Verification items for the finished model (mm, model axes). Face numbers are marked on the shaded views. A direction names the side the tool comes from. Round coordinates to 2 decimals unless told otherwise and drop trailing zeros. Write each loop counter-clockwise with the first axis right and the second up, starting at its lowest first coordinate (ties: lowest second). Pieces come first, ordered by that corner, then holes. Notation, with made-up numbers: M 54,-24 L 58,-24 A16 cw 58,3 Z; hole C 60,57.5 d1. An arc over 180 degrees is marked long. One line per question, with ' | ' between items.
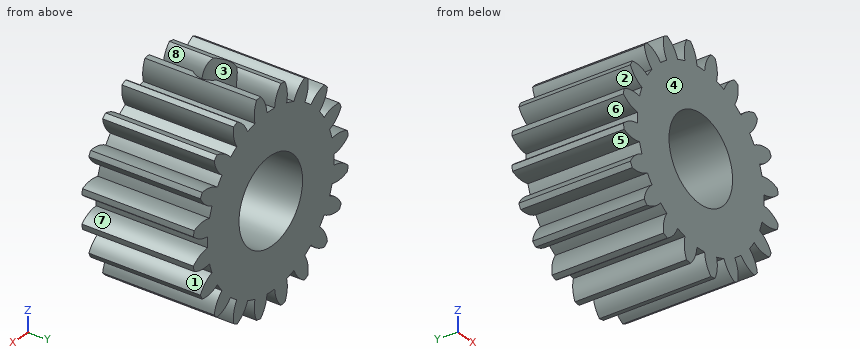
from build123d import *

# Parameters (mm, degrees)
SKETCH1_R                    = 11.684
BOSS_EXTRUDE1_DEPTH          = 12.7
F_3_8_0_375_DIAMETER_HOLE1_D = 9.525
CUT_EXTRUDE1_DEPTH           = 21.840386561
CIRPATTERN1_COUNT            = 20
F_10_32_TAPPED_HOLE2_REACH   = 30.849
F_10_32_TAPPED_HOLE2_BORE_R  = 2.0193


with BuildPart() as part:
    # Sketch1 → Boss-Extrude1 (new body)
    with BuildSketch(Plane(origin=(0, 0, 0), x_dir=(1, 0, 0), z_dir=(0, 1, 0))):
        with Locations(Location((0, 0, 0), (0, 0, 270))):
            Circle(SKETCH1_R)
    extrude(amount=BOSS_EXTRUDE1_DEPTH)

    # 3/8 (0.375) Diameter Hole1 (through all)
    with Locations(Plane(origin=(0, 12.7, 0), x_dir=(1, 0, 0), z_dir=(0, 1, 0))):
        with Locations((0, 0)):
            Hole(F_3_8_0_375_DIAMETER_HOLE1_D / 2)

    # Sketch6 → Cut-Extrude1 (cut, through all)
    with BuildSketch(Plane(origin=(0, 12.7, 0), x_dir=(1, 0, 0), z_dir=(0, 1, 0))):
        with BuildLine():
            ThreePointArc((-1.52506803, 11.58404176), (0, 11.684), (1.52506803, 11.58404176))
            ThreePointArc((1.52506803, 11.58404176), (0.859486594, 10.605826694), (0.578386073, 9.456528707))
            ThreePointArc((0.578386073, 9.456528707), (0, 9.4742), (-0.578386073, 9.456528707))
            ThreePointArc((-0.578386073, 9.456528707), (-0.859486594, 10.605826694), (-1.52506803, 11.58404176))
        make_face()
    cut_extrude1 = extrude(amount=-CUT_EXTRUDE1_DEPTH, mode=Mode.SUBTRACT)

    # CirPattern1: Cut-Extrude1 ×20 about axis
    cirpattern1_axis = Axis((0, 0, 0), (0, 1, 0))
    for i in range(1, CIRPATTERN1_COUNT):
        add(cut_extrude1.rotate(cirpattern1_axis, i * 360 / CIRPATTERN1_COUNT), mode=Mode.SUBTRACT)

    # #10-32 Tapped Hole2 bore → #10-32 Tapped Hole2 (cut, up to next)
    with BuildSketch(Plane.XY.offset(11.58404176), mode=Mode.PRIVATE) as f_10_32_tapped_hole2_sk1:
        with Locations((0, 6.35)):
            Circle(F_10_32_TAPPED_HOLE2_BORE_R)
    f_10_32_tapped_hole2_tool1 = extrude(f_10_32_tapped_hole2_sk1.sketch, amount=-F_10_32_TAPPED_HOLE2_REACH, mode=Mode.PRIVATE) & part.part
    add(f_10_32_tapped_hole2_tool1.solids().sort_by_distance((0, 6.35, 11.584042))[0], mode=Mode.SUBTRACT)


solid = part.part
1. Go/stop test with flat-tipped pins: P1, Ø10, axis at x = 2, z = -1, coming from the +Y side; P2, Ø5.5, axis at x = 0, y = 6.35, coming from the -Z side; P3, Ø4, axis at y = 2, z = 8, coming from the +X side; P4, Ø1, axis at y = 4.5, z = 6, coming from the -X side. Record where each tip stops, or that it passes through.
Results:
P1: stops at y = 12.7 | P2: stops at z = -11.58 | P3: stops at x = 8.48 | P4: stops at x = -10.31
2. Section check C-C, the plane z = -3. Record the cut outline in (x, y).
Results:
outline: M -8.99,0 L -3.7,0 L -3.7,12.7 L -8.99,12.7 Z; M 3.7,0 L 8.99,0 L 8.99,12.7 L 3.7,12.7 Z
3. Tool access check on the marked faces 5, 6, 7 and 8. Record the directions out of +Z, -Z, +X, -X, +Y, -Y that give a thin tool (end or side, any length) a straight path to the whole face; none if there is none.
Results:
face 5: +Y, -Y | face 6: -X, +Y, -Y | face 7: +X, +Y, -Y | face 8: +Z, +Y, -Y
4. Thickness scan on line 1 (Z direction, x = 0, y = 4); line 2 (X direction, y = 6.35, z = 9.5); line 3 (Z direction, x = -9.25, y = 6). Record the ranges inside material, lowest first.
Results:
line 1: z = -9.47 to -4.76, 4.76 to 9.47 | line 2: x = -5.6 to -3.84, -2.44 to -2.02, 2.02 to 2.44, 3.84 to 5.6 | line 3: z = -5.57 to -3.68, -2.39 to 2.39, 3.68 to 5.57
5. Mould release check, pull along X, two halves, no side actions. Record for the marked faces 1, 2, 3 and 4: pulls with the +X half, pulls with the -X half, needs draft (parallel to the pull), parting line crosses it, or undercut.
Results:
face 1: pulls with the +X half | face 2: pulls with the -X half | face 3: undercut | face 4: needs draft
6. Section check A-A, the plane x = 0. Record the cut outline in (y, z), then the cut area to 3 significant figures.
Results:
outline: M 0,-9.47 L 12.7,-9.47 L 12.7,-4.76 L 0,-4.76 Z; M 0,4.76 L 4.33,4.76 L 4.33,9.47 L 0,9.47 Z; M 8.37,4.76 L 12.7,4.76 L 12.7,9.47 L 8.37,9.47 Z | area: 101 mm2
7. Section check B-B, the plane z = 0. Record the cut outline in (x, y).
Results:
outline: M -9.47,0 L -4.76,0 L -4.76,12.7 L -9.47,12.7 Z; M 4.76,0 L 9.47,0 L 9.47,12.7 L 4.76,12.7 Z
